Could you check a few things on this model? Use its own coordinates, in mm. Face numbers are marked on the shaded views. A direction names the side the tool comes from. Coordinates: 2 decimals unless noted, no trailing zeros. Loops run counter-clockwise (first coordinate to the right, second up) from the corner with the lowest first, then second, coordinate; pieces in that order, holes last. Notation, with made-up numbers: M -4,-1.75 L 53,-1.75 A25 ccw 53,20.25 Z; hole C 14.25,84 d9. An arc over 180 degrees is marked long. Return JSON: item names as keys, results as strings. Group by question number.
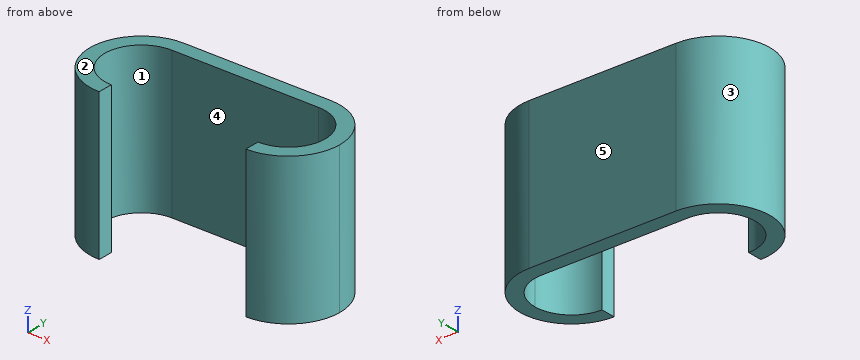
from build123d import *

# Parameters (mm, degrees)
F1_DEPTH = 25.4


with BuildPart() as f1:
    # F0 (on Top) → F1 (new body)
    with BuildSketch(Plane.XY):
        with BuildLine():
            ThreePointArc((-12.7, 8.89), (-21.59, 0), (-12.7, -8.89))
            Line((-12.7, -8.89), (-12.7, -6.35))
            ThreePointArc((-12.7, -6.35), (-19.05, 0), (-12.7, 6.35))
            Line((-12.7, 6.35), (-12.7, 8.89))
        make_face()
        with BuildLine():
            Line((-6.478296, 6.35), (6.478296, 6.35))
            ThreePointArc((6.478296, 6.35), (9.339896, 8.230541), (12.7, 8.89))
            Line((12.7, 8.89), (-12.7, 8.89))
            ThreePointArc((-12.7, 8.89), (-9.339896, 8.230541), (-6.478296, 6.35))
        make_face()
        with BuildLine():
            Line((6.478296, 6.35), (12.7, 6.35))
            Line((12.7, 6.35), (12.7, 8.89))
            ThreePointArc((12.7, 8.89), (9.339896, 8.230541), (6.478296, 6.35))
        make_face()
        with BuildLine():
            Line((-12.7, 6.35), (-6.478296, 6.35))
            ThreePointArc((-6.478296, 6.35), (-9.339896, 8.230541), (-12.7, 8.89))
            Line((-12.7, 8.89), (-12.7, 6.35))
        make_face()
        with BuildLine():
            ThreePointArc((19.05, 0), (17.190128, -4.490128), (12.7, -6.35))
            Line((12.7, -6.35), (12.7, -8.89))
            ThreePointArc((12.7, -8.89), (18.986179, -6.286179), (21.59, 0))
            ThreePointArc((21.59, 0), (18.986179, 6.286179), (12.7, 8.89))
            Line((12.7, 8.89), (12.7, 6.35))
            ThreePointArc((12.7, 6.35), (17.190128, 4.490128), (19.05, 0))
        make_face()
    extrude(amount=F1_DEPTH)


solid = f1.part
(1) If I drill on L1, parallel to Y at x = -4.5, z = 15.75; L2, parallel to Y at x = 13, z = 4; L3, parallel to X at y = 1, z = 14.25, over which ranges is the centre line in solid material (lowest first)? Write a range as [from, to].
(2) We'd pull the mould along X, two halves only. Please class the marked faces 1, 2 and 3: +X half, -X half, draft (parallel to the pull), parting line (faces both ways), or undercut.
(3) Imagine slicing it at C-C, the plane y = 2. Write out the boundary of the cut face in (x, z).
(4) Will these pins go through, and if not, where does the flat tip stop? P1, Ø1, axis at x = -16, z = 22, coming from the -Y side; P2, Ø6, axis at x = 14, y = 3, coming from the -Z side; P3, Ø2, axis at y = -7.5, z = 7.5, coming from the -X side; P4, Ø1, axis at x = 13.5, z = 17, coming from the -Y side.
(5) Imagine slicing it at D-D, the plane x = -2.5. Write out the boundary of the cut face in (y, z).
(6) Imagine slicing it at B-B, the plane x = -16. Write out the boundary of the cut face in (y, z).
(7) For the marked faces 4 and 5, which set-ups out of +Z, -Z, +X, -X, +Y, -Y let a thin tool reach every point of the face, with its end or its side?
(8) Imagine slicing it at A-A, the plane z = 23. Write out the boundary of the cut face in (x, y), then the cut area to 3 significant figures.
Checks:
{
 "1": {"L1": "[6.35, 8.89]", "L2": "[-8.88, -6.34], [6.34, 8.88]", "L3": "[-21.53, -18.97], [18.97, 21.53]"},
 "2": {"face 1": "undercut", "face 2": "draft", "face 3": "-X half"},
 "3": {"outline": "M -21.36,0 L -18.73,0 L -18.73,25.4 L -21.36,25.4 Z; M 18.73,0 L 21.36,0 L 21.36,25.4 L 18.73,25.4 Z"},
 "4": {"P1": "y = -8.44", "P2": "through", "P3": "x = -18.76", "P4": "y = -8.88"},
 "5": {"outline": "M 6.35,0 L 8.89,0 L 8.89,25.4 L 6.35,25.4 Z"},
 "6": {"outline": "M -8.25,0 L -5.43,0 L -5.43,25.4 L -8.25,25.4 Z; M 5.43,0 L 8.25,0 L 8.25,25.4 L 5.43,25.4 Z"},
 "7": {"face 4": "+Z, -Z, -Y", "face 5": "+Z, -Z, +X, -X, +Y"},
 "8": {"outline": "M -12.7,-8.89 L -12.7,-6.35 A6.35 cw -12.7,6.35 L 12.7,6.35 A6.35 cw 12.7,-6.35 L 12.7,-8.89 A8.89 ccw 21.59,0 A8.89 ccw 12.7,8.89 L -12.7,8.89 A8.89 ccw Z", "area": "186 mm²"}
}
